from build123d import *

# Parameters (mm, degrees)
EXTRUDE003_DEPTH  = 5
BOX025_W          = 13.75
BOX025_H          = 18.5
BOX025_DEPTH      = 5
CYLINDER031_R     = 4.1
CYLINDER031_DEPTH = 5
BOX024_W          = 18
BOX024_H          = 18.5
BOX024_DEPTH      = 5
ARRAY035_COUNT    = 3
TUBE016_R         = 60.5
TUBE016_R_2       = 59
TUBE016_DEPTH     = 11
TUBE017_R         = 61.5
TUBE017_R_2       = 60.5
TUBE017_DEPTH     = 15
TUBE024_R         = 55.25
TUBE024_R_2       = 51.75
TUBE024_DEPTH     = 5
TUBE025_R         = 51.9
TUBE025_R_2       = 49.4
TUBE025_DEPTH     = 15
TUBE015_R         = 59
TUBE015_R_2       = 55.25
TUBE015_DEPTH     = 15


with BuildPart() as cockpitrailconnectornutcutout:
    # Face003 → Extrude003 (new body)
    with BuildSketch(Plane(origin=(-40.5, 0, 500), x_dir=(0, 1, 0), z_dir=(0, 0, 1))):
        Polygon((0, -7.5), (6.495191, -3.75), (6.495191, 3.75), (0, 7.5), (-6.495191, 3.75), (-6.495191, -3.75), align=None)
    extrude(amount=-EXTRUDE003_DEPTH)


with BuildPart() as cockpitrailconnectornutanchor1:
    # Box025 → Box025 (new body)
    with BuildSketch(Plane(origin=(-51, -9.25, 495), x_dir=(1, 0, 0), z_dir=(0, 0, 1))):
        with Locations((6.875, 9.25)):
            Rectangle(BOX025_W, BOX025_H)
    extrude(amount=BOX025_DEPTH)

    # Cut059: cut CockpitRailConnectorNutCutout
    add(cockpitrailconnectornutcutout.part, mode=Mode.SUBTRACT)


with BuildPart() as cockpitrailconnectorrailcutter:
    # Cylinder031 → Cylinder031 (new body)
    with BuildSketch(Plane(origin=(-40.5, 0, 490), x_dir=(1, 0, 0), z_dir=(0, 0, 1))):
        Circle(CYLINDER031_R)
    extrude(amount=CYLINDER031_DEPTH)


with BuildPart() as cockpitrailconnectors:
    # Box024 → Box024 (new body)
    with BuildSketch(Plane(origin=(-49.5, -9.25, 490), x_dir=(1, 0, 0), z_dir=(0, 0, 1))):
        with Locations((9, 9.25)):
            Rectangle(BOX024_W, BOX024_H)
    extrude(amount=BOX024_DEPTH)

    # Cut058: cut CockpitRailConnectorRailCutter
    add(cockpitrailconnectorrailcutter.part, mode=Mode.SUBTRACT)

    # Fusion018: union CockpitRailConnectorNutAnchor1
    add(cockpitrailconnectornutanchor1.part)

    # Array035: CockpitRailConnectors ×3 about axis
    array035_axis = Axis((0, 0, 0), (0, 0, 1))


with BuildPart() as cockpitrailconnectors_1:
    add(cockpitrailconnectors.part)
    for i in range(1, ARRAY035_COUNT):
        add(cockpitrailconnectors.part.rotate(array035_axis, i * 360 / ARRAY035_COUNT))


with BuildPart() as cockpitmountcenter:
    # Tube016 → Tube016 (new body)
    with BuildSketch(Plane.XY):
        Circle(TUBE016_R)
        Circle(TUBE016_R_2, mode=Mode.SUBTRACT)
    extrude(amount=TUBE016_DEPTH)


with BuildPart() as cockpitmountouter:
    # Tube017 → Tube017 (new body)
    with BuildSketch(Plane.XY):
        Circle(TUBE017_R)
        Circle(TUBE017_R_2, mode=Mode.SUBTRACT)
    extrude(amount=TUBE017_DEPTH)


with BuildPart() as cockpitconnectorcenter:
    # Tube024 → Tube024 (new body)
    with BuildSketch(Plane.XY.offset(10)):
        Circle(TUBE024_R)
        Circle(TUBE024_R_2, mode=Mode.SUBTRACT)
    extrude(amount=TUBE024_DEPTH)


with BuildPart() as cockpitconnectorinner:
    # Tube025 → Tube025 (new body)
    with BuildSketch(Plane.XY):
        Circle(TUBE025_R)
        Circle(TUBE025_R_2, mode=Mode.SUBTRACT)
    extrude(amount=TUBE025_DEPTH)


with BuildPart() as cockpitglassmount2:
    # Tube015 → Tube015 (new body)
    with BuildSketch(Plane.XY):
        Circle(TUBE015_R)
        Circle(TUBE015_R_2, mode=Mode.SUBTRACT)
    extrude(amount=TUBE015_DEPTH)

    # Fusion007: union CockpitMountCenter, CockpitMountOuter, CockpitConnectorCenter, CockpitConnectorInner
    add(cockpitmountcenter.part)
    add(cockpitmountouter.part)
    add(cockpitconnectorcenter.part)
    add(cockpitconnectorinner.part)


with BuildPart() as cockpitglassmount2_1:
    # Fusion007 placement: moved
    add(cockpitglassmount2.part.moved(Location((0, 0, 490))))

    # Fusion019: union CockpitRailConnectors
    add(cockpitrailconnectors_1.part)


solid = cockpitglassmount2_1.part
Input: part model. Units: mm. Frame: model coordinates. A direction names the side the tool comes from. Give positions to 0.01 mm unless a question says otherwise; leave off trailing zeros. Loops run counter-clockwise (first coordinate to the right, second up) from the corner with the lowest first, then second, coordinate; pieces in that order, holes last. Notation, with made-up numbers: M 44.25,31.25 L 66.25,31.25 A11 cw 66.25,35.25 Z; hole C 69,32 d2. An arc over 180 degrees is marked long. Use one line per item in the form item = value.
1. First-contact query: pin 1 (1.5 mm diameter, centred on y = 3.5, z = 493, fed in from +X); pin 2 (15 mm diameter, centred on x = 15, y = 28, fed in from +Z); pin 3 (2.5 mm diameter, centred on x = -42.5, z = 496.5, fed in from -Y); pin 4 (9.5 mm diameter, centred on x = 20.25, y = 35.07, fed in from -Z). Flat tips, straight axial feed; report the tip coordinate or a pass-through.
Numbers:
pin_1 = 61.44
pin_2 = 495
pin_3 = -45.61
pin_4 = 490
2. Section query B-B, the plane x = 0. Return the cut outline in (y, z), and give its area (3 significant figures).
Numbers:
outline = M -61.5,490 L -55.25,490 L -55.25,500 L -51.9,500 L -51.9,490 L -49.4,490 L -49.4,505 L -59,505 L -59,501 L -60.5,501 L -60.5,505 L -61.5,505 Z; M 49.4,490 L 51.9,490 L 51.9,500 L 55.25,500 L 55.25,490 L 61.5,490 L 61.5,505 L 60.5,505 L 60.5,501 L 59,501 L 59,505 L 49.4,505 Z
area = 284 mm²
3. Reachability of faces 1 (the face through (-13, -48, 505)), 2 (the face through (-31.5, 0, 492)), 3 (the face through (-41, 6.495, 498)) from +Z, -Z, +X, -X, +Y, -Y: full face, straight path, thin tool, end or side. Return the list, or none.
Numbers:
face_1 = +Z, +X, -X, +Y, -Y
face_2 = +Z, -Z
face_3 = +Z
4. Section query C-C, the plane y = -12.5. Return the cut outline in (x, z).
Numbers:
outline = M -60.22,490 L -53.82,490 L -53.82,500 L -50.37,500 L -50.37,490 L -47.79,490 L -47.79,505 L -57.66,505 L -57.66,501 L -59.19,501 L -59.19,505 L -60.22,505 Z; M 47.79,490 L 50.37,490 L 50.37,500 L 53.82,500 L 53.82,490 L 60.22,490 L 60.22,505 L 59.19,505 L 59.19,501 L 57.66,501 L 57.66,505 L 47.79,505 Z
5. Pull-direction query (X, two-part tool) for faces 4 (the face through (-50.4, 23.1, 490)), 5 (the face through (29.023, 31.769, 494.93)); classes: released by +X, released by -X, zero draft, split by the parting line, or undercut.
Numbers:
face_4 = zero draft
face_5 = undercut
6. Section query A-A, the plane z = 498.25. Count the separate pieces of the cut face and the enclosed holes in it, and give its area (3 significant figures).
Numbers:
separate_pieces = 2
enclosed_holes = 2
area = 3,400 mm²
7. Line query: L1, parallel to Y at x = 0, z = 501.5; L2, parallel to Y at x = 0, z = 496; L3, parallel to X at y = 17, z = 496. Output: solid intervals per line, ascending.
Numbers:
L1 = -61.5 to -60.5, -59 to -49.4, 49.4 to 59, 60.5 to 61.5
L2 = -61.5 to -55.25, -51.9 to -49.4, 49.4 to 51.9, 55.25 to 61.5
L3 = -59.1 to -52.57, -49.04 to -46.38, 46.38 to 49.04, 52.57 to 59.1
